Build history of the part. All positions in model axes, mm. A direction names the side the tool comes from. Coordinates: 2 decimals unless noted, no trailing zeros. Order: outer loops, then holes, each group sorted by start corner. A loop starts at its lowest first (then second) coordinate and runs counter-clockwise, first axis right, second up. Notation, with made-up numbers: (-7, 69) - (43, 69) arc R13 ccw to (43, 77) - close; hole circle Ø8 at (34.5, 55.25). An arc over 180 degrees is marked (long way). One line per item, written item: value.
from build123d import *

# Parameters (mm, degrees)
SKETCH2_W           = 26
SKETCH2_H           = 11.2
BOSS_EXTRUDE1_DEPTH = 20
SKETCH6_W           = 14
SKETCH6_H           = 2.4
CUT_EXTRUDE1_DEPTH  = 20
SKETCH7_W           = 10.08
SKETCH7_H           = 4.9
CUT_EXTRUDE2_DEPTH  = 15
SKETCH8_W           = 19
SKETCH8_H           = 1.78
CUT_EXTRUDE3_DEPTH  = 16
SKETCH9_W           = 15.8
SKETCH9_H           = 2.12
CUT_EXTRUDE4_DEPTH  = 15
SKETCH10_W          = 3
SKETCH10_H          = 2
CUT_EXTRUDE5_DEPTH  = 15
CUT_REVOLVE3_ANGLE  = 180
SKETCH15_W          = 12
SKETCH15_H          = 6
BOSS_EXTRUDE2_DEPTH = 10
SKETCH16_W          = 12
SKETCH16_H          = 6
BOSS_EXTRUDE3_DEPTH = 10
SKETCH17_R          = 2
CUT_EXTRUDE6_DEPTH  = 12
SKETCH18_R          = 2
CUT_EXTRUDE7_DEPTH  = 12
SKETCH19_W          = 7.8
SKETCH19_H          = 20
BOSS_EXTRUDE4_DEPTH = 15
SKETCH20_W          = 20
SKETCH20_H          = 12
BOSS_EXTRUDE5_DEPTH = 10
SKETCH21_R          = 4.05
CUT_EXTRUDE8_DEPTH  = 18
SKETCH22_R          = 1.5
CUT_EXTRUDE9_DEPTH  = 5


with BuildPart() as part:
    # Sketch2 → Boss-Extrude1 (new body)
    with BuildSketch(Plane.XY):
        Rectangle(SKETCH2_W, SKETCH2_H)
    extrude(amount=BOSS_EXTRUDE1_DEPTH)

    # Sketch6 → Cut-Extrude1 (cut)
    with BuildSketch(Plane.XY.offset(20)):
        with Locations((0, -4.4)):
            Rectangle(SKETCH6_W, SKETCH6_H)
    extrude(amount=-CUT_EXTRUDE1_DEPTH, mode=Mode.SUBTRACT)

    # Sketch7 → Cut-Extrude2 (cut)
    with BuildSketch(Plane.XY.offset(20)):
        with Locations((0, -0.75)):
            Rectangle(SKETCH7_W, SKETCH7_H)
    extrude(amount=-CUT_EXTRUDE2_DEPTH, mode=Mode.SUBTRACT)

    # Sketch8 → Cut-Extrude3 (cut)
    with BuildSketch(Plane.XY.offset(20)):
        with Locations((2.3, 2.59)):
            Rectangle(SKETCH8_W, SKETCH8_H)
    extrude(amount=-CUT_EXTRUDE3_DEPTH, mode=Mode.SUBTRACT)

    # Sketch9 → Cut-Extrude4 (cut)
    with BuildSketch(Plane.XY.offset(20)):
        with Locations((2.7, 4.54)):
            Rectangle(SKETCH9_W, SKETCH9_H)
    extrude(amount=-CUT_EXTRUDE4_DEPTH, mode=Mode.SUBTRACT)

    # Sketch10 → Cut-Extrude5 (cut)
    with BuildSketch(Plane.XY.offset(20)):
        with Locations((9.1, 0.7)):
            Rectangle(SKETCH10_W, SKETCH10_H)
    extrude(amount=-CUT_EXTRUDE5_DEPTH, mode=Mode.SUBTRACT)

    # Sketch11 → Cut-Revolve3 (revolve, cut)
    with BuildSketch(Plane.XZ.offset(5.6)):
        with BuildLine():
            Line((-11.55, 5), (-8.45, 5))
            ThreePointArc((-8.45, 5), (-10, 6.55), (-11.55, 5))
        make_face()
    revolve(axis=Axis((-11.55, -5.6, 5), (-1, 0, 0)), revolution_arc=CUT_REVOLVE3_ANGLE, mode=Mode.SUBTRACT)

    # Sketch12 → Revolve2 (revolve)
    with BuildSketch(Plane.XZ.offset(5.6)):
        with BuildLine():
            Line((-11.5, 15), (-8.5, 15))
            ThreePointArc((-8.5, 15), (-10, 13.5), (-11.5, 15))
        make_face()
    revolve(axis=Axis((-11.5, -5.6, 15), (1, 0, 0)))

    # Sketch14 → Cut-Revolve4 (revolve, cut)
    with BuildSketch(Plane.XZ.offset(5.6)):
        with BuildLine():
            Line((8.45, 15), (11.55, 15))
            ThreePointArc((11.55, 15), (10, 13.45), (8.45, 15))
        make_face()
    revolve(axis=Axis((8.45, -5.6, 15), (1, 0, 0)), mode=Mode.SUBTRACT)

    # Sketch13 → Revolve3 (revolve)
    with BuildSketch(Plane.XZ.offset(5.6)):
        with BuildLine():
            Line((8.5, 5), (11.5, 5))
            ThreePointArc((11.5, 5), (10, 6.5), (8.5, 5))
        make_face()
    revolve(axis=Axis((8.5, -5.6, 5), (1, 0, 0)))

    # Sketch15 → Boss-Extrude2 (add)
    with BuildSketch(Plane.ZY.offset(13)):
        with Locations((6, -2.6)):
            Rectangle(SKETCH15_W, SKETCH15_H)
    extrude(amount=BOSS_EXTRUDE2_DEPTH)

    # Sketch16 → Boss-Extrude3 (add)
    with BuildSketch(Plane(origin=(13, 0, 0), x_dir=(0, 0, -1), z_dir=(1, 0, 0))):
        with Locations((-6, -2.6)):
            Rectangle(SKETCH16_W, SKETCH16_H)
    extrude(amount=BOSS_EXTRUDE3_DEPTH)

    # Sketch17 → Cut-Extrude6 (cut)
    with BuildSketch(Plane.XZ.offset(5.6)):
        with Locations(Location((-18, 6, 0), (0, 0, 270))):
            Circle(SKETCH17_R)
    extrude(amount=-CUT_EXTRUDE6_DEPTH, mode=Mode.SUBTRACT)

    # Sketch18 → Cut-Extrude7 (cut)
    with BuildSketch(Plane.XZ.offset(5.6)):
        with Locations(Location((18, 6, 0), (0, 0, 270))):
            Circle(SKETCH18_R)
    extrude(amount=-CUT_EXTRUDE7_DEPTH, mode=Mode.SUBTRACT)

    # Sketch19 → Boss-Extrude4 (add)
    with BuildSketch(Plane(origin=(0, 5.6, 0), x_dir=(1, 0, 0), z_dir=(0, 1, 0))):
        with Locations((-9.1, -10)):
            Rectangle(SKETCH19_W, SKETCH19_H)
    extrude(amount=BOSS_EXTRUDE4_DEPTH)

    # Sketch20 → Boss-Extrude5 (add)
    with BuildSketch(Plane.ZY.offset(13)):
        with Locations((10, 14.6)):
            Rectangle(SKETCH20_W, SKETCH20_H)
    extrude(amount=BOSS_EXTRUDE5_DEPTH)

    # Sketch21 → Cut-Extrude8 (cut)
    with BuildSketch(Plane.XY.offset(20)):
        with Locations((-17, 14.6)):
            Circle(SKETCH21_R)
    extrude(amount=-CUT_EXTRUDE8_DEPTH, mode=Mode.SUBTRACT)

    # Sketch22 → Cut-Extrude9 (cut)
    with BuildSketch(Plane.ZY.offset(23)):
        with Locations(Location((11, 14.6, 0), (0, 0, 270))):
            Circle(SKETCH22_R)
    extrude(amount=-CUT_EXTRUDE9_DEPTH, mode=Mode.SUBTRACT)


solid = part.part
1. Band-saw the part on C-C, the plane z = 14.25. Count the separate pieces of the cut face and the enclosed holes in it, and give its area (3 significant figures).
Values found:
separate pieces: 2
enclosed holes: 1
area: 320 mm2
2. Band-saw the part on A-A, the plane x = 18. Give the cut face in (y, z).
Values found:
outline: (-5.6, 0) - (0.4, 0) - (0.4, 4) - (-5.6, 4) - close; (-5.6, 8) - (0.4, 8) - (0.4, 12) - (-5.6, 12) - close
3. 3-axis set-ups, long thin cutter, end or side, ignore diameter. For faces 4 (the face through (-7, -4, 10)), 5 (the face through (9, -0.3, 13)), 6 (the face through (18, -3, 12)), 7 (the face through (-18, -3, 12)): which of +Z, -Z, +X, -X, +Y, -Y reach the whole face in a straight line?
Values found:
face 4: +Z, -Z, -Y
face 5: +Z, +Y
face 6: +Z, +X, +Y, -Y
face 7: +Z, -X, -Y
4. Flat gauge pins, fed straight in: P1, Ø8, axis at x = 16.5, z = 5.5, coming from the +Y side; P2, Ø0.5, axis at x = 4.5, y = 3, coming from the +Z side; P3, Ø2, axis at y = 7.5, z = 13, coming from the +X side. Where does each tip first touch, or does it go through?
Values found:
P1: stops at y = 5.6
P2: stops at z = 4
P3: stops at x = -5.2
5. Probe line 1 along X through (y, z) = (0.5, 18.5); line 2 along X through (y, z) = (-2.15, 6); line 3 along X through (y, z) = (-3.4, 6). List the from-to ranges inside material, lowest first.
Values found:
line 1: x = -13 to -5.04, 5.04 to 7.6, 10.6 to 13
line 2: x = -23 to -20, -16 to -5.04, 5.04 to 16, 20 to 23
line 3: x = -23 to -20, -16 to -7, 7 to 16, 20 to 23
6. Band-saw the part on B-B, the plane y = 14.6. Give the cut face in (x, z).
Values found:
outline: (-23, 0) - (-5.2, 0) - (-5.2, 20) - (-12.95, 20) - (-12.95, 2) - (-21.05, 2) - (-21.05, 9.5) - (-23, 9.5) - close; (-23, 12.5) - (-21.05, 12.5) - (-21.05, 20) - (-23, 20) - close
7. Two-plate mould, pull along Y, no slides. Class faces 1 (the face through (5.2, 5.6, 4.8)), 2 (the face through (7.6, 1, 13)), 3 (the face through (-21.9, 16.1, 11.07)): pulls with the +Y half, pulls with the -Y half, needs draft (parallel to the pull), parting line crosses it, or undercut.
Values found:
face 1: pulls with the +Y half
face 2: needs draft
face 3: undercut
